CAD build for the part. Positions are in the model's coordinates, mm. A direction names the side the tool comes from. Round coordinates to 2 decimals unless told otherwise and drop trailing zeros. Order: outer loops, then holes, each group sorted by start corner. A loop starts at its lowest first (then second) coordinate and runs counter-clockwise, first axis right, second up. Notation, with made-up numbers: M 21,52 L 65,52 A23 cw 65,67 Z; hole C 29.25,-11 d8. An arc over 180 degrees is marked long. Answer as a JSON object with one key per item and string values.
```python
from build123d import *

# Parameters (mm, degrees)
BOSS_EXTRUDE1_DEPTH = 6
FILLET1_R           = 2
SKETCH2_R           = 16
BOSS_EXTRUDE2_DEPTH = 2
CHAMFER1_SIZE       = 1
SKETCH3_R           = 3.5
CUT_EXTRUDE1_DEPTH  = 37.800135869


with BuildPart() as part:
    # Sketch1 → Boss-Extrude1 (new body)
    with BuildSketch(Plane(origin=(0, 0, 0), x_dir=(1, 0, 0), z_dir=(0, 1, 0))):
        with BuildLine():
            Line((-18, 22.5), (24, 22.5))
            ThreePointArc((24, 22.5), (26.828427125, 21.328427125), (28, 18.5))
            Line((28, 18.5), (28, -18.5))
            ThreePointArc((28, -18.5), (26.828427125, -21.328427125), (24, -22.5))
            Line((24, -22.5), (-18, -22.5))
            ThreePointArc((-18, -22.5), (-20.828427125, -21.328427125), (-22, -18.5))
            Line((-22, -18.5), (-22, 18.5))
            ThreePointArc((-22, 18.5), (-20.828427125, 21.328427125), (-18, 22.5))
        make_face()
    extrude(amount=BOSS_EXTRUDE1_DEPTH)

    # Fillet1
    fillet1_edges = [part.edges().sort_by_distance(p)[0] for p in [
        (-20.828427125, 6, -21.328427125),
        (-22, 6, 0),
        (-20.828427125, 6, 21.328427125),
        (3, 6, 22.5),
        (26.828427125, 6, 21.328427125),
        (28, 6, 0),
        (26.828427125, 6, -21.328427125),
        (3, 6, -22.5),
    ]]
    fillet(fillet1_edges, radius=FILLET1_R)

    # Sketch2 → Boss-Extrude2 (add)
    with BuildSketch(Plane.XZ):
        with Locations(Location((0, 0, 0), (0, 0, 270))):
            Circle(SKETCH2_R)
    extrude(amount=BOSS_EXTRUDE2_DEPTH)

    # Chamfer1
    chamfer1_edges = [part.edges().sort_by_distance(p)[0] for p in [
        (0, -2, 16),
    ]]
    chamfer(chamfer1_edges, length=CHAMFER1_SIZE)

    # Sketch3 → Cut-Extrude1 (cut, through all)
    with BuildSketch(Plane(origin=(0, 6, 0), x_dir=(1, 0, 0), z_dir=(0, 1, 0))):
        with Locations(Location((-16.263455967, 16.263455967, 0), (0, 0, 270))):
            Circle(SKETCH3_R)
        with Locations(Location((16.263455967, 16.263455967, 0), (0, 0, 270))):
            Circle(SKETCH3_R)
        with Locations(Location((16.263455967, -16.263455967, 0), (0, 0, 270))):
            Circle(SKETCH3_R)
        with Locations(Location((-16.263455967, -16.263455967, 0), (0, 0, 270))):
            Circle(SKETCH3_R)
    extrude(amount=-CUT_EXTRUDE1_DEPTH, mode=Mode.SUBTRACT)


solid = part.part
```
Item 1: Saw through at A-A on x = 0. List the corners of the cut face in (y, z).
Worked answers:
{"outline": "M -2,-15 L -1,-16 L 0,-16 L 0,-22.5 L 4,-22.5 A2 ccw 6,-20.5 L 6,20.5 A2 ccw 4,22.5 L 0,22.5 L 0,16 L -1,16 L -2,15 Z"}
Item 2: Two-plate mould, pull along Z, no slides. Class faces 1 (the flat face through (3, 2, 22.5)), 2 (the cylindrical face through (-18.393, 3.042, -19.041)), 3 (the cylindrical face through (12.847, 3.042, -17.022)), 4 (the flat face through (-22, 2, 0)): released by +Z, released by -Z, zero draft, split by the parting line, or undercut.
Worked answers:
{"face 1": "released by +Z", "face 2": "undercut", "face 3": "undercut", "face 4": "zero draft"}
Item 3: Saw through at D-D on z = 0. List the corners of the cut face in (x, y).
Worked answers:
{"outline": "M -22,0 L -16,0 L -16,-1 L -15,-2 L 15,-2 L 16,-1 L 16,0 L 28,0 L 28,4 A2 ccw 26,6 L -20,6 A2 ccw -22,4 Z"}
Item 4: Saw through at B-B on z = -17. List the corners of the cut face in (x, y).
Worked answers:
{"outline": "M -22,0 L -19.69,0 L -19.69,6 L -20,6 A2 ccw -22,4 Z; M -12.84,0 L 12.84,0 L 12.84,6 L -12.84,6 Z; M 19.69,0 L 28,0 L 28,4 A2 ccw 26,6 L 19.69,6 Z"}
Item 5: Drop a flat-ended pin along its axis: pin 1 Ø2 at (x, z) = (4.5, 16.5) entering from -Y. Give the stop position or say it passes through.
Worked answers:
{"pin 1": "stops at y = 0"}
Item 6: Saw through at C-C on x = 19. List the corners of the cut face in (y, z), and give its area (3 significant figures).
Worked answers:
{"outline": "M 0,-22.5 L 4,-22.5 A2 ccw 6,-20.5 L 6,-18.45 L 0,-18.45 Z; M 0,-14.08 L 6,-14.08 L 6,14.08 L 0,14.08 Z; M 0,18.45 L 6,18.45 L 6,20.5 A2 ccw 4,22.5 L 0,22.5 Z", "area": "216 mm2"}
Item 7: Wall check: line 1 along Z through (x, y) = (-16.5, 2); line 2 along Z through (x, y) = (14, 5.5); line 3 along Y through (x, z) = (-2.5, 18). Give the ranges that are in metal, low to high. Write a range as [from, to].
Worked answers:
{"line 1": "z = [-22.5, -19.76], [-12.77, 12.77], [19.76, 22.5]", "line 2": "z = [-21.82, -18.93], [-13.59, 13.59], [18.93, 21.82]", "line 3": "y = [0, 6]"}
Item 8: 3-axis set-ups, long thin cutter, end or side, ignore diameter. For faces 5 (the flat face through (14, 0, -10)), 6 (the cylindrical face through (27.43, 5.4, 0.26)): which of +Z, -Z, +X, -X, +Y, -Y reach the whole face in a straight line?
Worked answers:
{"face 5": "-Y", "face 6": "+Z, -Z, +X, +Y"}
